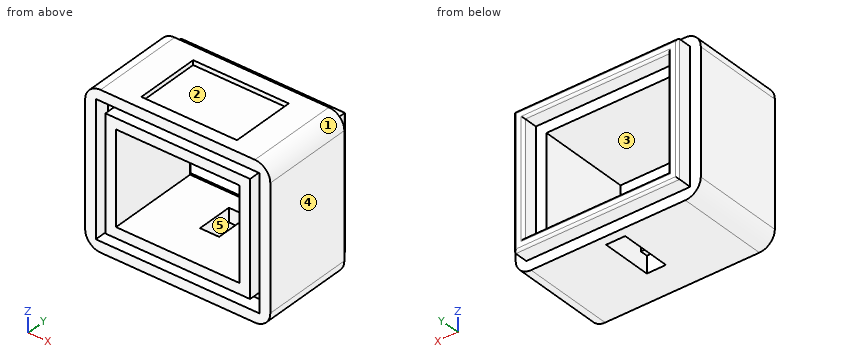
from build123d import *

# Parameters (mm, degrees)
BOSS_EXTRUDE1_DEPTH      = 50
BOSS_EXTRUDE1_DEPTH_BACK = 10
SKETCH1_W                = 120
SKETCH1_H                = 100
FILLET1_R                = 10
SKETCH2_W                = 80
SKETCH2_H                = 60
CUT_EXTRUDE1_DEPTH       = 99.488578018
SKETCH3_W                = 106.2
SKETCH3_H                = 86.2
SKETCH3_W_2              = 93.8
SKETCH3_H_2              = 73.8
CUT_EXTRUDE2_DEPTH       = 10
SKETCH4_W                = 106.2
SKETCH4_H                = 86.2
SKETCH4_W_2              = 93.8
SKETCH4_H_2              = 73.8
BOSS_EXTRUDE2_DEPTH      = 10
FILLET2_R                = 1.5
SKETCH5_W                = 12.4
SKETCH5_H                = 33
CUT_EXTRUDE3_DEPTH       = 11
SKETCH10_W               = 62
SKETCH10_H               = 42
CUT_EXTRUDE7_DEPTH       = 3
CUT_EXTRUDE8_DEPTH       = 20


with BuildPart() as part:
    # Sketch1 → Boss-Extrude1 (new, two sides: drawn at the far end of the back side and taken through both)
    with BuildSketch(Plane(origin=(0, 0, 0), x_dir=(1, 0, 0), z_dir=(0, 1, 0)).offset(-BOSS_EXTRUDE1_DEPTH_BACK)):
        Rectangle(SKETCH1_W, SKETCH1_H)
    extrude(amount=BOSS_EXTRUDE1_DEPTH + BOSS_EXTRUDE1_DEPTH_BACK)

    # Fillet1
    fillet1_edges = [part.edges().sort_by_distance(p)[0] for p in [
        (-60, 20, -50),
        (60, 20, -50),
        (60, 20, 50),
        (-60, 20, 50),
    ]]
    fillet(fillet1_edges, radius=FILLET1_R)

    # Sketch2 → Cut-Extrude1 (cut, through all)
    with BuildSketch(Plane(origin=(0, 50, 0), x_dir=(1, 0, 0), z_dir=(0, 1, 0))):
        Rectangle(SKETCH2_W, SKETCH2_H)
    extrude(amount=-CUT_EXTRUDE1_DEPTH, mode=Mode.SUBTRACT)

    # Sketch3 → Cut-Extrude2 (cut)
    with BuildSketch(Plane.XZ.offset(10)):
        Rectangle(SKETCH3_W, SKETCH3_H)
        Rectangle(SKETCH3_W_2, SKETCH3_H_2, mode=Mode.SUBTRACT)
    extrude(amount=-CUT_EXTRUDE2_DEPTH, mode=Mode.SUBTRACT)

    # Sketch4 → Boss-Extrude2 (add)
    with BuildSketch(Plane(origin=(0, 50, 0), x_dir=(1, 0, 0), z_dir=(0, 1, 0))):
        Rectangle(SKETCH4_W, SKETCH4_H)
        Rectangle(SKETCH4_W_2, SKETCH4_H_2, mode=Mode.SUBTRACT)
    extrude(amount=BOSS_EXTRUDE2_DEPTH)

    # Fillet2
    fillet2_edges = [part.edges().sort_by_distance(p)[0] for p in [
        (-46.9, 60, 0),
        (0, 60, 36.9),
        (46.9, 60, 0),
        (0, 60, -36.9),
        (0, 60, -43.1),
        (-53.1, 60, 0),
        (0, 60, 43.1),
        (53.1, 60, 0),
    ]]
    fillet(fillet2_edges, radius=FILLET2_R)

    # Sketch5 → Cut-Extrude3 (cut)
    with BuildSketch(Plane(origin=(0, 0, -50), x_dir=(-1, 0, 0), z_dir=(0, 0, -1))):
        with Locations((0, 27.5)):
            Rectangle(SKETCH5_W, SKETCH5_H)
    extrude(amount=-CUT_EXTRUDE3_DEPTH, mode=Mode.SUBTRACT)

    # Sketch10 → Cut-Extrude7 (cut)
    with BuildSketch(Plane.XY.offset(50)):
        with Locations((1, 19)):
            Rectangle(SKETCH10_W, SKETCH10_H)
    extrude(amount=-CUT_EXTRUDE7_DEPTH, mode=Mode.SUBTRACT)

    # Sketch9 → Cut-Extrude8 (cut)
    with BuildSketch(Plane(origin=(0, 0, -50), x_dir=(-1, 0, 0), z_dir=(0, 0, -1))):
        Polygon((-6.2, 27.5), (-6.2, 39.2), (6.2, 39.2), (6.2, 15.8), (-6.2, 15.8), align=None)
    extrude(amount=-CUT_EXTRUDE8_DEPTH, mode=Mode.SUBTRACT)


solid = part.part
Model file for the job. Use its own axes, mm. Face numbers are marked on the shaded views. A direction names the side the tool comes from. Coordinates: 2 decimals unless noted, no trailing zeros. Loops run counter-clockwise (first coordinate to the right, second up) from the corner with the lowest first, then second, coordinate; pieces in that order, holes last. Notation, with made-up numbers: (87.5, 79.5) -> (97.5, 79.5) arc R16 ccw to (97.5, 92.5) -> close; hole circle Ø11 at (49, -17). An arc over 180 degrees is marked (long way). Use one line per item in the form item = value. Start each with the question number.
(1) Tool access for the marked faces 3, 4 and 5: list every direction of +Z, -Z, +X, -X, +Y, -Y with a clear straight run to the whole face (end or side of a thin tool).
(2) Cut at D-D on x = -43. Give the cut face in (y, z), and give its area (3 significant figures).
(3) Cut at C-C on y = 46. Give the cut face in (x, z), and give its area (3 significant figures).
(4) Pull direction Y, two halves, no side cores. Call the marked faces 1 and 2: pulls with the +Y half, pulls with the -Y half, needs draft (parallel to the pull), parting line crosses it, or undercut.
(5) Flat gauge pins, fed straight in: pin 1 (1.5 mm diameter, centred on y = 13.5, z = 49, fed in from -X); pin 2 (7 mm diameter, centred on x = 7, y = 56, fed in from +Z); pin 3 (5 mm diameter, centred on x = 27.5, y = 9.5, fed in from +Z). Where does each tip first touch, or does it go through?
(6) Cut at A-A on z = -12. Give the cut face in (x, y), and give its area (3 significant figures).
(7) Probe probe 1 along Z at (x, y) = (-16.5, -3); probe 2 along X at (y, z) = (-3.5, -15); probe 3 along X at (y, z) = (49, -1). List the from-to ranges inside material, lowest first. Write a range as from..to.
Values:
q1.face_3 = +Y, -Y
q1.face_4 = +Z, -Z, +X, +Y, -Y
q1.face_5 = -Z
q2.outline = (-10, -50) -> (50, -50) -> (50, -43.1) -> (58.5, -43.1) arc R1.5 ccw to (60, -41.6) -> (60, -38.4) arc R1.5 ccw to (58.5, -36.9) -> (50, -36.9) -> (50, 36.9) -> (58.5, 36.9) arc R1.5 ccw to (60, 38.4) -> (60, 41.6) arc R1.5 ccw to (58.5, 43.1) -> (50, 43.1) -> (50, 50) -> (-10, 50) -> (-10, 43.1) -> (0, 43.1) -> (0, 36.9) -> (-10, 36.9) -> (-10, -36.9) -> (0, -36.9) -> (0, -43.1) -> (-10, -43.1) -> close
q2.area = 6,000 mm2
q3.outline = (-60, -40) arc R10 ccw to (-50, -50) -> (50, -50) arc R10 ccw to (60, -40) -> (60, 40) arc R10 ccw to (50, 50) -> (-50, 50) arc R10 ccw to (-60, 40) -> close; hole (-40, -30) -> (40, -30) -> (40, 30) -> (-40, 30) -> close
q3.area = 7,110 mm2
q4.face_1 = needs draft
q4.face_2 = undercut
q5.pin_1 = -55.65
q5.pin_2 = 43.1
q5.pin_3 = 47
q6.outline = (-60, -10) -> (-53.1, -10) -> (-53.1, 0) -> (-46.9, 0) -> (-46.9, -10) -> (-40, -10) -> (-40, 50) -> (-46.9, 50) -> (-46.9, 58.5) arc R1.5 ccw to (-48.4, 60) -> (-51.6, 60) arc R1.5 ccw to (-53.1, 58.5) -> (-53.1, 50) -> (-60, 50) -> close; (40, -10) -> (46.9, -10) -> (46.9, 0) -> (53.1, 0) -> (53.1, -10) -> (60, -10) -> (60, 50) -> (53.1, 50) -> (53.1, 58.5) arc R1.5 ccw to (51.6, 60) -> (48.4, 60) arc R1.5 ccw to (46.9, 58.5) -> (46.9, 50) -> (40, 50) -> close
q6.area = 2,400 mm2
q7.probe_1 = -50..-43.1, -36.9..-30, 30..36.9, 43.1..50
q7.probe_2 = -60..-53.1, -46.9..-40, 40..46.9, 53.1..60
q7.probe_3 = -60..-40, 40..60
